The model under review builds one solid part; all positions refer to its coordinate system, in mm. Face numbers are marked on the shaded views. A direction names the side the tool comes from. Coordinates: 2 decimals unless noted, no trailing zeros. Order: outer loops, then holes, each group sorted by start corner. A loop starts at its lowest first (then second) coordinate and runs counter-clockwise, first axis right, second up. Notation, with made-up numbers: (37.5, -29.5) - (74.5, -29.5) arc R10 cw to (74.5, -17.5) - close; hole circle Ø2 at (-31.75, 76). An arc over 180 degrees is marked (long way). Answer in a Markdown table with one row per item.
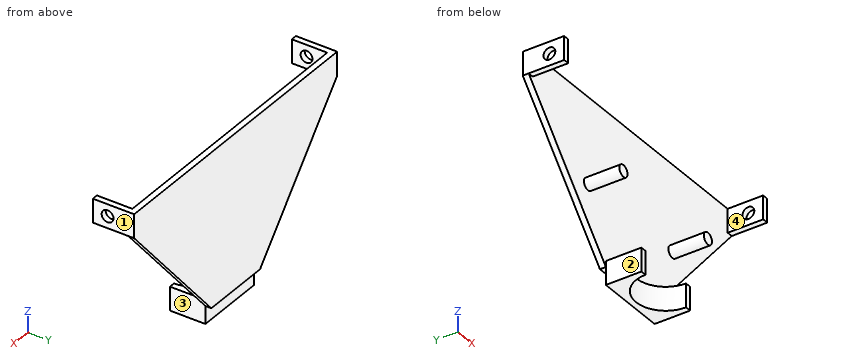
Solid Edge part; units mm, degrees
sketch "Sketch1" plane through (0, 0, 0) normal (0, -1, 0) x (1, 0, 0)
  line L0 (110.6916, 92.473) -> (110.6916, 112.473)
  line L1 (110.6916, 112.473) -> (-139.3084, 112.473)
  line L2 (-139.3084, 112.473) -> (-139.3084, 92.473)
  line L3 (-139.3084, 92.473) -> (-44.3084, -17.527)
  line L4 (-44.3084, -17.527) -> (15.6916, -17.527)
  line L5 (15.6916, -17.527) -> (110.6916, 92.473)
  dimension "D1" = 139.3084
  dimension "D2" = 110.6916
  dimension "D3" = 44.3084
  dimension "D4" = 110.6916
extrude "ExtrudedProtrusion_1" add sketch "Sketch1" against normal blind 5
sketch "Sketch2" plane through (10.6916, 0, 44.973) normal (0, -1, 0) x (1, 0, 0)
  line L0 (95, 47.5) -> (100, 47.5)
  line L1 (100, 47.5) -> (100, 67.5)
  line L2 (100, 67.5) -> (95, 67.5)
  line L3 (95, 67.5) -> (95, 47.5)
  line L4 (-55, -77.5) -> (5, -77.5)
  line L5 (5, -77.5) -> (5, -57.5)
  line L6 (5, -57.5) -> (-55, -57.5)
  line L7 (-55, -57.5) -> (-55, -77.5)
  circle A0 centre (-77, -5.5) radius 5
  circle A1 centre (27, -5.5) radius 5
  line L8 (-150, 47.5) -> (-145, 47.5)
  line L9 (-145, 47.5) -> (-145, 67.5)
  line L10 (-145, 67.5) -> (-150, 67.5)
  line L11 (-150, 67.5) -> (-150, 47.5)
  dimension "D1" = 150
  dimension "D2" = 145
  dimension "D3" = 145
  dimension "D4" = 100
  dimension "D5" = 95
  dimension "D6" = 55
  dimension "D7" = 55
extrude "Protrusion1" add sketch "Sketch2" along normal blind 30
sketch "Sketch3" plane through (-14.3084, -50, 24.202) normal (0, 0, 1) x (0, 1, 0)
  circle A0 centre (20, 0) radius 25
extrude "Cutout1" cut sketch "Sketch3" against normal through all
sketch "Sketch4" plane through (160.6916, -12.5, 96.702) normal (1, 0, 0) x (0, 1, 0)
  circle A0 centre (-5, 5.7698) radius 5
extrude "Cutout2" cut sketch "Sketch4" against normal through all
Item 1: We need section C-C, the plane z = 51. Write out the cut boundary in (x, y), then the cut area to 3 significant figures.
Check values:
| item | result |
|---|---|
| outline | (-103.49, 0) - (74.87, 0) - (74.87, 5) - (-103.49, 5) - close |
| area | 892 mm^2 |
Item 2: To check wall thickness, follow line 1 (Z direction, x = 108.05, y = -17.5); line 2 (Z direction, x = -136, y = -17); line 3 (X direction, y = -17.5, z = 97). State the ranges of each line that lie inside material, in increasing order. Write a range as from..to.
Check values:
| item | result |
|---|---|
| line 1 | 92.47..97.47, 107.47..112.47 |
| line 2 | 92.47..97.5, 107.45..112.47 |
| line 3 | -139.31..-134.31, 105.69..110.69 |
Item 3: We need section A-A, the plane y = -17.5. Write out the cut boundary in (x, z).
Check values:
| item | result |
|---|---|
| outline | (-139.31, 92.47) - (-134.31, 92.47) - (-134.31, 97.47) - (-139.31, 97.47) - close; (-139.31, 107.47) - (-134.31, 107.47) - (-134.31, 112.47) - (-139.31, 112.47) - close; circle Ø10 at (-66.31, 39.47); (-44.31, -32.53) - (-35.96, -32.53) - (-35.96, -12.53) - (-44.31, -12.53) - close; (7.34, -32.53) - (15.69, -32.53) - (15.69, -12.53) - (7.34, -12.53) - close; circle Ø10 at (37.69, 39.47); (105.69, 92.47) - (110.69, 92.47) - (110.69, 97.47) - (105.69, 97.47) - close; (105.69, 107.47) - (110.69, 107.47) - (110.69, 112.47) - (105.69, 112.47) - close |
Item 4: We need section B-B, the plane x = -17. Write out the cut boundary in (y, z).
Check values:
| item | result |
|---|---|
| outline | (-5.15, -32.53) - (0, -32.53) - (0, -17.53) - (5, -17.53) - (5, 112.47) - (0, 112.47) - (0, -12.53) - (-5.15, -12.53) - close |
Item 5: Tool access review of the marked faces 1, 2, 3 and 4: name each direction out of +Z, -Z, +X, -X, +Y, -Y from which nothing blocks a thin tool from reaching the whole face with its end or side.
Check values:
| item | result |
|---|---|
| face 1 | +Z, -Z, +X, +Y, -Y |
| face 2 | +Z, -Z, -X, -Y |
| face 3 | +Z, -Z, +X, -Y |
| face 4 | +Z, -Z, -Y |
Item 6: We need section D-D, the plane x = -120. Write out the cut boundary in (y, z), then the cut area to 3 significant figures.
Check values:
| item | result |
|---|---|
| outline | (0, 70.12) - (5, 70.12) - (5, 112.47) - (0, 112.47) - close |
| area | 212 mm^2 |
Item 7: Clearance check with flat-ended pins moving along their axes: pin 1 Ø10 at (y, z) = (-20.5, -20.5) entering from +X; pin 2 Ø1 at (y, z) = (1, 27) entering from -X; pin 3 Ø4 at (x, y) = (34.5, 0.5) entering from -Z. State where each tip first meets the part, or that it passes through.
Check values:
| item | result |
|---|---|
| pin 1 | x = 15.69 |
| pin 2 | x = -83.2 |
| pin 3 | z = 1.94 |
